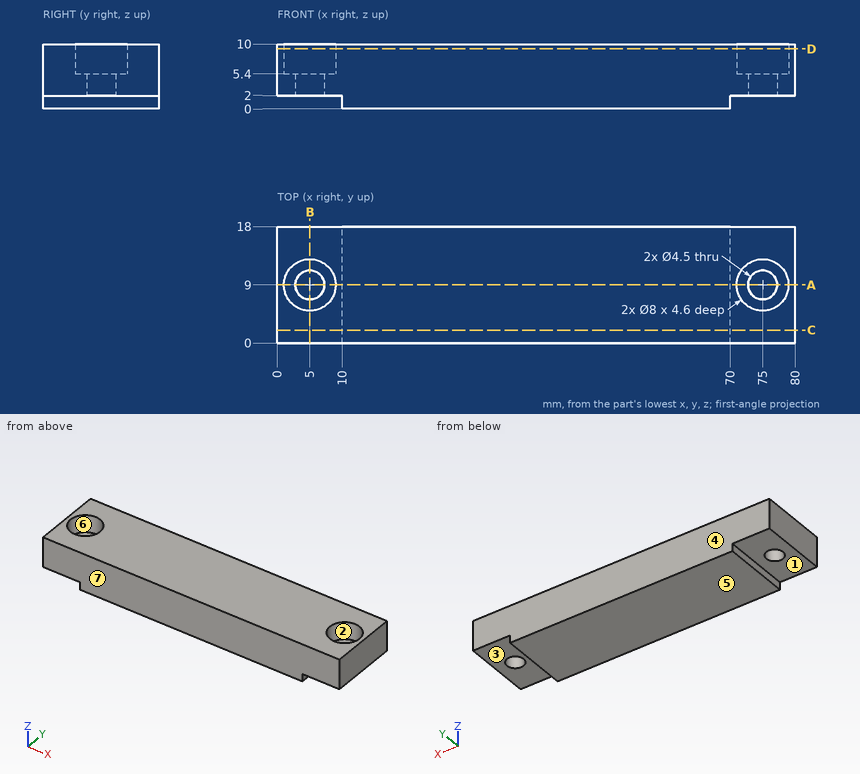
Design review of the part shown in the three views and the two pictorial views. Dimensions are in mm from the part's minimum x, y and z. A direction names the side the tool comes from. Coordinates: 2 decimals unless noted, no trailing zeros. Order: outer loops, then holes, each group sorted by start corner. A loop starts at its lowest first (then second) coordinate and runs counter-clockwise, first axis right, second up.
Item 1: Take a section at A-A, the plane y = 9. Write out the cut boundary in (x, z), then the cut area to 3 significant figures.
Item 2: Take a section at D-D, the plane z = 9.25. Write out the cut boundary in (x, y), then the cut area to 3 significant figures.
Item 3: Take a section at B-B, the plane x = 5. Write out the cut boundary in (y, z).
Item 4: The part is to be moulded in two halves that separate along Y. For the marked faces 5, 6 and 7, say which applies: pulls with the +Y half, pulls with the -Y half, needs draft (parallel to the pull), parting line crosses it, or undercut.
Item 5: For the marked faces 1, 2, 3 and 4, list the 3-axis set-ups (+Z, -Z, +X, -X, +Y, -Y) from which the entire face can be reached by the end or side of a thin tool; tool diameter is ignored.
Item 6: For pin 1 Ø6 at (x, y) = (5, 9) entering from +Z; pin 2 Ø1.6 at (y, z) = (10, 0.5) entering from -X; pin 3 Ø5 at (x, y) = (75, 9) entering from -Z; pin 4 Ø2.5 at (x, y) = (5, 9) entering from +Z, all flat-tipped, find the tip position at first contact; note any pin that passes through.
Item 7: Take a section at C-C, the plane y = 2. Write out the cut boundary in (x, z), then the cut area to 3 significant figures.
Item 8: For line 1 (X direction, y = 9, z = 6.85); line 2 (Y direction, x = 5, z = 7.35); line 3 (Y direction, x = 5, z = 4.6), list the stretches that pass through material, from the lowest coordinate up.
The answers:
1. outline: (0, 2) - (2.75, 2) - (2.75, 5.4) - (1, 5.4) - (1, 10) - (0, 10) - close; (7.25, 2) - (10, 2) - (10, 0) - (70, 0) - (70, 2) - (72.75, 2) - (72.75, 5.4) - (71, 5.4) - (71, 10) - (9, 10) - (9, 5.4) - (7.25, 5.4) - close; (77.25, 2) - (80, 2) - (80, 10) - (79, 10) - (79, 5.4) - (77.25, 5.4) - close
1. area: 656 mm2
2. outline: (0, 0) - (80, 0) - (80, 18) - (0, 18) - close; hole circle Ø8 at (5, 9); hole circle Ø8 at (75, 9)
2. area: 1,340 mm2
3. outline: (0, 2) - (6.75, 2) - (6.75, 5.4) - (5, 5.4) - (5, 10) - (0, 10) - close; (11.25, 2) - (18, 2) - (18, 10) - (13, 10) - (13, 5.4) - (11.25, 5.4) - close
4. face 5: needs draft
4. face 6: undercut
4. face 7: pulls with the -Y half
5. face 1: -Z, -X, +Y, -Y
5. face 2: +Z
5. face 3: -Z, +X, +Y, -Y
5. face 4: +Z, -Z, +X, -X, +Y
6. pin 1: stops at z = 5.4
6. pin 2: stops at x = 10
6. pin 3: stops at z = 2
6. pin 4: passes through
7. outline: (0, 2) - (10, 2) - (10, 0) - (70, 0) - (70, 2) - (80, 2) - (80, 10) - (0, 10) - close
7. area: 760 mm2
8. line 1: x = 0 to 1, 9 to 71, 79 to 80
8. line 2: y = 0 to 5, 13 to 18
8. line 3: y = 0 to 6.75, 11.25 to 18
